Read the model definition and answer for the solid it produces. Units are mm, in the model's axes. A direction names the side the tool comes from. Give positions to 0.01 mm unless a question says otherwise; leave off trailing zeros. Write each loop counter-clockwise with the first axis right and the second up, starting at its lowest first coordinate (ties: lowest second). Pieces come first, ordered by that corner, then holes. Notation, with made-up numbers: (-2, -5) - (31, -5) arc R18 cw to (31, 26) - close; hole circle Ø10 at (75.25, 6.5). An arc over 180 degrees is marked (long way). Answer as CSV lines item,"result".
```python
from build123d import *

# Parameters (mm, degrees)
SKETCH1_W           = 75
SKETCH1_H           = 80
BOSS_EXTRUDE1_DEPTH = 3
SKETCH2_W           = 75
SKETCH2_H           = 3
BOSS_EXTRUDE2_DEPTH = 75
SKETCH5_R           = 2.5
BOSS_EXTRUDE3_DEPTH = 3.1
SKETCH8_R           = 2.5


with BuildPart() as part:
    # Sketch1 → Boss-Extrude1 (new body)
    with BuildSketch(Plane.XY):
        with Locations((-37.5, 40)):
            Rectangle(SKETCH1_W, SKETCH1_H)
    extrude(amount=BOSS_EXTRUDE1_DEPTH)

    # Sketch2 → Boss-Extrude2 (add)
    with BuildSketch(Plane.XY.offset(3)):
        with Locations((-37.5, 1.5)):
            Rectangle(SKETCH2_W, SKETCH2_H)
    extrude(amount=BOSS_EXTRUDE2_DEPTH)

    # Sketch5 → Boss-Extrude3 (add)
    with BuildSketch(Plane.XY.offset(3)):
        with Locations((-37.5, 65)):
            Circle(SKETCH5_R)
    extrude(amount=-BOSS_EXTRUDE3_DEPTH)

    # Sweep1: sweep along a path in Sketch7
    with BuildLine(Plane(origin=(0, 0, 0), x_dir=(0, 0, -1), z_dir=(1, 0, 0))) as sweep1_path:
        Line((0, 64.541389485), (50, 64.541389485))
        ThreePointArc((50, 64.541389485), (53.535533906, 63.076923391), (55, 59.541389485))
        Line((55, 59.541389485), (55, 19.541389485))
        ThreePointArc((55, 19.541389485), (53.535533906, 16.005855579), (50, 14.541389485))
        Line((50, 14.541389485), (0, 14.541389485))
    # Sketch8 → Sweep1 (sweep)
    with BuildSketch(Plane(origin=(0, 0, -0.1), x_dir=(-1, 0, 0), z_dir=(0, 0, -1))):
        with Locations((37.5, 65)):
            Circle(SKETCH8_R)
    sweep(path=sweep1_path.line)


solid = part.part
```
(1) Find the intervals of material crossed by L1, parallel to Y at x = -35, z = 55.5; L2, parallel to Z at x = -39, y = 59, in increasing order.
Worked out:
L1,"y = 0 to 3"
L2,"z = -57.46 to -53.46, 0 to 3"
(2) A cutting plane is placed at D-D (z = 26.5). Write down the section's boundary in (x, y).
Worked out:
outline,"(-75, 0) - (0, 0) - (0, 3) - (-75, 3) - close"
(3) A cutting plane is placed at C-C (y = 31). Write down the section's boundary in (x, z), and give its area (3 significant figures).
Worked out:
outline,"(-75, 0) - (0, 0) - (0, 3) - (-75, 3) - close; circle Ø5 at (-37.5, -55.46)"
area,"245 mm^2"
(4) Each of these flat-tipped pins is pushed along its axis until it touches: P1, Ø22.5, axis at x = -55, y = 39, coming from the -Z side; P2, Ø6, axis at x = -66, z = 63.5, coming from the +Y side; P3, Ø12, axis at x = -31.5, z = -42.5, coming from the -Y side. Where does it stop, or does it pass through?
Worked out:
P1,"stops at z = 0"
P2,"stops at y = 3"
P3,"stops at y = 11.58"
(5) The mould has two halves that part along Z. Classify faces 1 (the cylindrical face through (-39.81, 15.04, -24.65)), 2 (the flat face through (-38, 42, 3)), 3 (the flat face through (-38, 3, 40)): +Z half, -Z half, draft (parallel to the pull), parting line (faces both ways), or undercut.
Worked out:
face 1,"undercut"
face 2,"+Z half"
face 3,"draft"
(6) A cutting plane is placed at B-B (x = -21.5). Write down the section's boundary in (y, z).
Worked out:
outline,"(0, 0) - (80, 0) - (80, 3) - (3, 3) - (3, 78) - (0, 78) - close"
(7) For faces 4 (the flat face through (-38, 2, 78)), 5 (the cylindrical face through (-38.84, 39.26, -57.57)), determine the directions among +Z, -Z, +X, -X, +Y, -Y from which every point of the face is accessible in a straight line to the end or side of a thin tool.
Worked out:
face 4,"+Z, +X, -X, +Y, -Y"
face 5,"none"
(8) A cutting plane is placed at A-A (x = -37.5). Write down the section's boundary in (y, z), and give its area (3 significant figures).
Worked out:
outline,"(0, 0) - (11.58, 0) - (11.58, -50) arc R7.96 ccw to (19.54, -57.96) - (59.54, -57.96) arc R7.96 ccw to (67.5, -50) - (67.5, 0) - (80, 0) - (80, 3) - (3, 3) - (3, 78) - (0, 78) - close; hole (16.58, -50) arc R2.96 ccw to (19.54, -52.96) - (59.54, -52.96) arc R2.96 ccw to (62.5, -50) - (62.5, 0) - (16.58, 0) - close"
area,"1,250 mm^2"
